Input: dimensioned drawing with shaded views. Units: mm. Origin: part minimum x, y, z. A direction names the side the tool comes from. Round coordinates to 2 decimals unless told otherwise and drop trailing zeros. Loops run counter-clockwise (first coordinate to the right, second up) from the corner with the lowest first, then second, coordinate; pieces in that order, holes last. Notation, with made-up numbers: (80, 34) - (133, 34) arc R31 cw to (133, 68) - close; hole circle Ø9 at (21.5, -37.75). An arc over 180 degrees is marked (long way). Use CSV: the item, a comma, the result in double quotes. Start each with the question number.
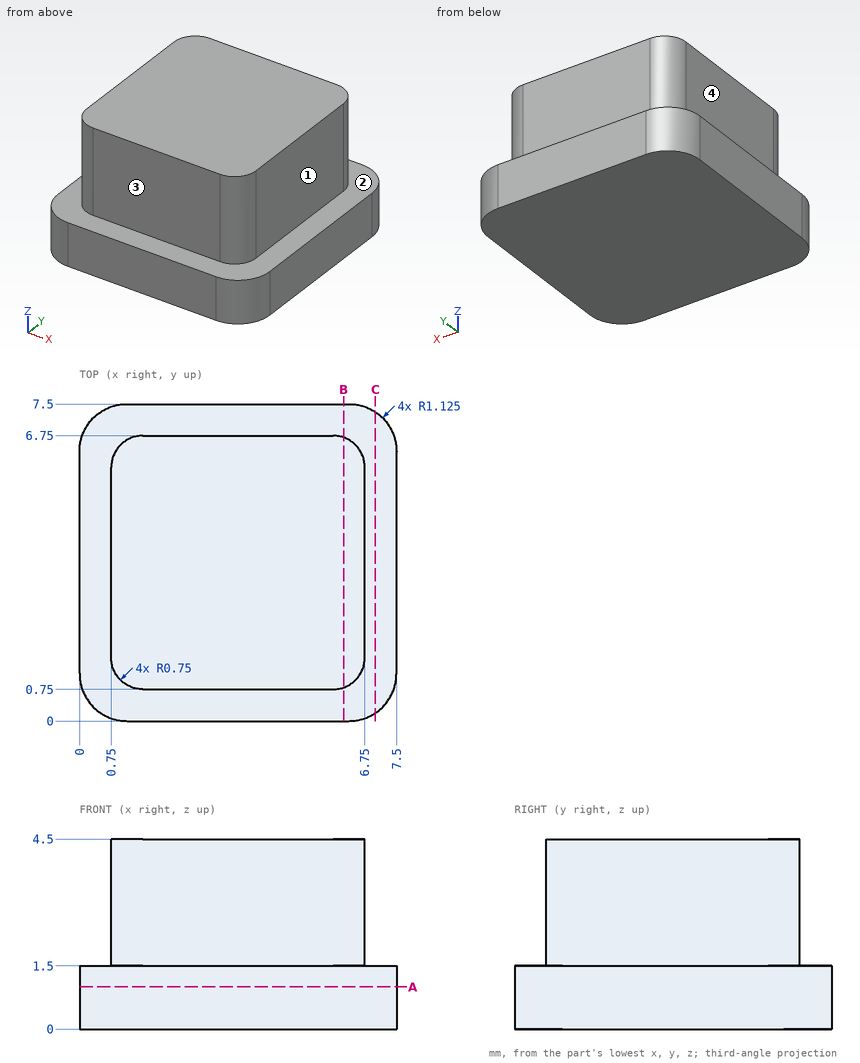
1. Section query A-A on z = 1. Return the cut outline in (x, y) (3 decimals).
2. Line query: line 1 along Y through (x, z) = (2.75, 3); line 2 along Z through (x, y) = (0.5, 0.5). Output: solid intervals per line, ascending.
3. Section query B-B on x = 6.25. Return the cut outline in (y, z), and give its area (3 significant figures).
4. Section query C-C on x = 7. Return the cut outline in (y, z).
5. Contact query for flat-ended pins moving along their axis: P1, Ø0.9, axis at y = 4.5, z = 3, coming from the -X side; P2, Ø2.5, axis at x = 4, z = 3.5, coming from the -Y side; P3, Ø2.5, axis at x = 5, z = 3.5, coming from the +Y side. Output: stop coordinate, or through.
6. Reachability of the marked faces 1, 2, 3 and 4 from +Z, -Z, +X, -X, +Y, -Y: full face, straight path, thin tool, end or side. Return the list, or none.
Values:
1,outline,"(0, 1.125) arc R1.125 ccw to (1.125, 0) - (6.375, 0) arc R1.125 ccw to (7.5, 1.125) - (7.5, 6.375) arc R1.125 ccw to (6.375, 7.5) - (1.125, 7.5) arc R1.125 ccw to (0, 6.375) - close"
2,line 1,"y = 0.75 to 6.75"
2,line 2,"z = 0 to 1.5"
3,outline,"(0, 0) - (7.5, 0) - (7.5, 1.5) - (6.71, 1.5) - (6.71, 4.5) - (0.79, 4.5) - (0.79, 1.5) - (0, 1.5) - close"
3,area,"29.0 mm^2"
4,outline,"(0.19, 0) - (7.31, 0) - (7.31, 1.5) - (0.19, 1.5) - close"
5,P1,"stops at x = 0.75"
5,P2,"stops at y = 0.75"
5,P3,"stops at y = 6.75"
6,face 1,"+Z, +X, +Y, -Y"
6,face 2,"+Z"
6,face 3,"+Z, +X, -X, -Y"
6,face 4,"+Z, -X, +Y, -Y"
